Autodesk Inventor part; units mm, degrees
ref_plane "YZ Plane" through (0, 0, 0) normal (1, 0, 0) x (0, 1, 0)
ref_plane "XZ Plane" through (0, 0, 0) normal (0, 1, 0) x (-1, 0, 0)
ref_plane "XY Plane" through (0, 0, 0) normal (0, 0, 1) x (1, 0, 0)
sketch "Sketch1" plane through (0, 0, 0) normal (0, 0, 1) x (1, 0, 0)
  line L0 (-35, 40) -> (35, 40)
  line L1 (40, 35) -> (40, -35)
  line L2 (35, -40) -> (-35, -40)
  line L3 (-40, -35) -> (-40, 35)
  line L4 (-40, 40) -> (40, -40) construction
  line L5 (40, 40) -> (-40, -40) construction
  arc A0 (-35, 40) -> (-40, 35) centre (-35, 35) ccw
  arc A1 (40, 35) -> (35, 40) centre (35, 35) ccw
  arc A2 (35, -40) -> (40, -35) centre (35, -35) ccw
  arc A3 (-40, -35) -> (-35, -40) centre (-35, -35) ccw
  line L6 (35, 38) -> (-35, 38)
  arc A4 (-35, 38) -> (-38, 35) centre (-35, 35) ccw
  line L7 (-38, 35) -> (-38, -35)
  arc A5 (-38, -35) -> (-35, -38) centre (-35, -35) ccw
  line L8 (-35, -38) -> (35, -38)
  arc A6 (35, -38) -> (38, -35) centre (35, -35) ccw
  line L9 (38, -35) -> (38, 35)
  arc A7 (38, 35) -> (35, 38) centre (35, 35) ccw
  point P0 (0, 0)
  dimension "d0" = 80
  dimension "d1" = 5
  dimension "d2" = 2
extrude "Extrusion1" add sketch "Sketch1" along normal blind 260
sketch "Sketch2" plane through (0, 0, 0) normal (0, 1, 0) x (-1, 0, 0)
  line L0 (40, 0) -> (40, 260)
  line L1 (-40, 0) -> (-40, 260)
  line L2 (40, 260) -> (-40, 260)
  line L3 (40, 260) -> (-40, 138.8577)
  point P0 (0, 0)
  dimension "d5" = 123.44
extrude "Extrusion2" cut sketch "Sketch2" along normal through all both and the other way through all
properties part number "MSC 903 BASE TUBE"
Geometry: final body of the model. Coordinates: model frame, mm. A direction names the side the tool comes from. Give positions to 0.01 mm unless a question says otherwise; leave off trailing zeros. Write each loop counter-clockwise with the first axis right and the second up, starting at its lowest first coordinate (ties: lowest second). Pieces come first, ordered by that corner, then holes.
1. Section query B-B, the plane x = -6. Return loops of the section in (y, z).
2. Reachability of faces 4 (the flat face through (0, -38, 96)), 5 (the flat face through (0, -40, 96)) from +Z, -Z, +X, -X, +Y, -Y: full face, straight path, thin tool, end or side. Return the list, or none.
3. Section query C-C, the plane z = 112.5. Return loops of the section in (x, y), then the cut area to 3 significant figures.
4. Line query: probe 1 along Y at (x, z) = (13, 25); probe 2 along X at (y, z) = (34.5, 165.5). Output: solid intervals per line, ascending.
5. Section query D-D, the plane z = 219. Return loops of the section in (x, y), then the cut area to 3 significant figures.
6. Draft query along X for faces 1 (the flat face through (-40, 0, 128)), 2 (the flat face through (38, 0, 70)), 3 (the cylindrical face through (39, -38, 72)). Return one class per face: released by +X, released by -X, zero draft, split by the parting line, or undercut.
7. Pin query (flat end, axial travel): P1, Ø4, axis at y = -9, z = 189.5, coming from the +X side. Return the tip coordinate at first contact, or that it passes through.
8. Section query A-A, the plane y = 1. Return loops of the section in (x, z).
Computed:
1. outline: (-40, 0) - (-38, 0) - (-38, 208.51) - (-40, 208.51) - close; (38, 0) - (40, 0) - (40, 208.51) - (38, 208.51) - close
2. face 4: +Z, -Z
2. face 5: +Z, -Z, +X, -X, -Y
3. outline: (-40, -35) arc R5 ccw to (-35, -40) - (35, -40) arc R5 ccw to (40, -35) - (40, 35) arc R5 ccw to (35, 40) - (-35, 40) arc R5 ccw to (-40, 35) - close; hole (-38, -35) arc R3 ccw to (-35, -38) - (35, -38) arc R3 ccw to (38, -35) - (38, 35) arc R3 ccw to (35, 38) - (-35, 38) arc R3 ccw to (-38, 35) - close
3. area: 610 mm2
4. probe 1: y = -40 to -38, 38 to 40
4. probe 2: x = -40 to -38
5. outline: (-40, -35) arc R5 ccw to (-35, -40) - (-12.92, -40) - (-12.92, -38) - (-35, -38) arc R3 cw to (-38, -35) - (-38, 35) arc R3 cw to (-35, 38) - (-12.92, 38) - (-12.92, 40) - (-35, 40) arc R5 ccw to (-40, 35) - close
5. area: 253 mm2
6. face 1: released by -X
6. face 2: undercut
6. face 3: released by +X
7. P1: stops at x = -38
8. outline: (-40, 0) - (-38, 0) - (-38, 256.97) - (-40, 260) - close; (38, 0) - (40, 0) - (40, 138.86) - (38, 141.89) - close
